The drawing under review shows one solid part. Ordinate dimensions are in mm from its lowest x, y, z. A direction names the side the tool comes from. Coordinates: 2 decimals unless noted, no trailing zeros. Order: outer loops, then holes, each group sorted by start corner. A loop starts at its lowest first (then second) coordinate and runs counter-clockwise, first axis right, second up. Notation, with made-up numbers: M 3.5,66.5 L 36.5,66.5 A23 ccw 36.5,102.5 Z; hole C 57.5,11.25 d1. An arc over 180 degrees is marked long. Answer as a JSON object with one key per item and string values.
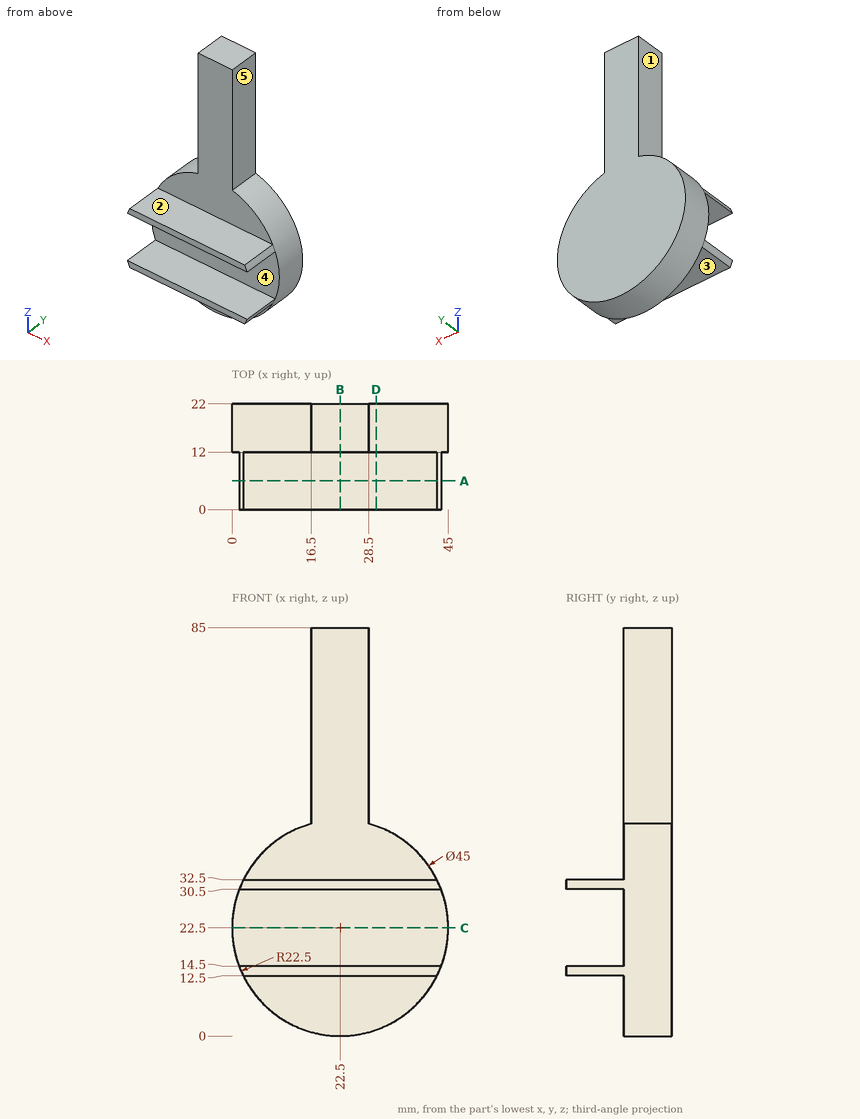
1) Tool access review of the marked faces 1, 2, 3, 4 and 5: name each direction out of +Z, -Z, +X, -X, +Y, -Y from which nothing blocks a thin tool from reaching the whole face with its end or side.
Taken from the geometry:
{"face 1": "+Z, -X, +Y, -Y", "face 2": "+Z, +X, -X, -Y", "face 3": "-Z, +X, -X, -Y", "face 4": "+X, -X, -Y", "face 5": "+Z, +X, +Y, -Y"}
2) Add section C-C (z = 22.5). State the section outline as (x, y) points, and give its area (3 significant figures).
Taken from the geometry:
{"outline": "M 0,12 L 45,12 L 45,22 L 0,22 Z", "area": "450 mm2"}
3) To check wall thickness, follow L1, parallel to Z at x = 17, y = 6.25; L2, parallel to Y at x = 27, z = 7.5; L3, parallel to X at y = 21, z = 61. State the ranges of each line that lie inside material, in increasing order.
Taken from the geometry:
{"L1": "z = 12.5 to 14.5, 30.5 to 32.5", "L2": "y = 12 to 22", "L3": "x = 16.5 to 28.5"}
4) Add section A-A (y = 6). State the section outline as (x, z) points.
Taken from the geometry:
{"outline": "M 1.47,14.5 A22.5 ccw 2.34,12.5 L 42.66,12.5 A22.5 ccw 43.53,14.5 Z; M 1.47,30.5 L 43.53,30.5 A22.5 ccw 42.66,32.5 L 2.34,32.5 A22.5 ccw Z"}
5) Add section B-B (x = 22.5). State the section outline as (y, z) points, and give its area (3 significant figures).
Taken from the geometry:
{"outline": "M 0,12.5 L 12,12.5 L 12,0 L 22,0 L 22,85 L 12,85 L 12,32.5 L 0,32.5 L 0,30.5 L 12,30.5 L 12,14.5 L 0,14.5 Z", "area": "898 mm2"}
6) Add section D-D (x = 30). State the section outline as (y, z) points, and give its area (3 significant figures).
Taken from the geometry:
{"outline": "M 0,12.5 L 12,12.5 L 12,1.29 L 22,1.29 L 22,43.71 L 12,43.71 L 12,32.5 L 0,32.5 L 0,30.5 L 12,30.5 L 12,14.5 L 0,14.5 Z", "area": "472 mm2"}
7) Insertion check: pin 1 Ø9.5 at (x, y) = (13.5, 3.5) entering from -Z; pin 2 Ø8 at (y, z) = (7, 31.5) entering from +X; pin 3 Ø11 at (y, z) = (16, 60.5) entering from +X; pin 4 Ø13 at (x, y) = (19, 7.5) entering from +Z. Each pin has a flat end and moves straight along its axis. Give the tip position at first contact, or say it passes through.
Taken from the geometry:
{"pin 1": "stops at z = 12.5", "pin 2": "stops at x = 43.53", "pin 3": "stops at x = 28.5", "pin 4": "stops at z = 85"}
